Model file for the job. Use its own axes, mm. Face numbers are marked on the shaded views. A direction names the side the tool comes from. Round coordinates to 2 decimals unless told otherwise and drop trailing zeros. Loops run counter-clockwise (first coordinate to the right, second up) from the corner with the lowest first, then second, coordinate; pieces in that order, holes last. Notation, with made-up numbers: M 64.5,39 L 105.5,39 A15 ccw 105.5,64 Z; hole C 34.25,25.5 d8. An arc over 180 degrees is marked long. Use a Markdown table: item, result. Add a question column.
Item 1: Saw through at A-A on z = 1.5. Write the cut outline in (x, y), then the cut area to 3 significant figures.
Item 2: Wall check: L1, parallel to Z at x = -16.5, y = 11; L2, parallel to X at y = -15, z = 12.5; L3, parallel to X at y = -8, z = 24.5. Give the ranges that are in metal, low to high. Write a range as from..to.
Item 3: Tool access for the marked faces 1, 2 and 3: list every direction of +Z, -Z, +X, -X, +Y, -Y with a clear straight run to the whole face (end or side of a thin tool).
Item 4: Saw through at C-C on x = 0. Write the cut outline in (y, z), then the cut area to 3 significant figures.
Item 5: Pin check, flat tips, straight feed: P1, Ø8, axis at x = -2, y = -15, coming from the +Z side; P2, Ø4, axis at x = -23.5, z = 15.5, coming from the +Y side; P3, Ø2, axis at x = 1, z = 6, coming from the +Y side. Stop position of each tip, or through.
Item 6: Saw through at D-D on y = -4. Write the cut outline in (x, z).
Item 7: Two-plate mould, pull along X, no slides. Class the marked faces 4, 5, 6 and 7: +X half, -X half, draft (parallel to the pull), parting line (faces both ways), or undercut.
Item 8: Saw through at B-B on y = 15. Write the cut outline in (x, z).
```python
from build123d import *

# Parameters (mm, degrees)
F1_DEPTH = 6.604
F3_DEPTH = 19.05
F4_DEPTH = 25.4


with BuildPart() as f1:
    # F0 (on Top) → F1 (new body)
    with BuildSketch(Plane.XY):
        with BuildLine():
            ThreePointArc((31.75, 12.954), (29.9645229381, 17.2645229381), (25.654, 19.05))
            Line((25.654, 19.05), (-25.654, 19.05))
            ThreePointArc((-25.654, 19.05), (-29.9645229381, 17.2645229381), (-31.75, 12.954))
            Line((-31.75, 12.954), (-31.75, -19.05))
            Line((-31.75, -19.05), (31.75, -19.05))
            Line((31.75, -19.05), (31.75, 12.954))
        make_face()
    extrude(amount=F1_DEPTH)

    # F2 (on face) → F3 (join)
    with BuildSketch(Plane.XY.offset(6.604)):
        with BuildLine():
            Line((-25.4, -19.05), (-18.796, -19.05))
            Line((-18.796, -19.05), (-18.796, -8.7467487901))
            Line((-18.796, -8.7467487901), (0, -8.7467487901))
            Line((0, -8.7467487901), (18.796, -8.7467487901))
            Line((18.796, -8.7467487901), (18.796, -19.05))
            Line((18.796, -19.05), (25.4, -19.05))
            Line((25.4, -19.05), (25.4, 0))
            Line((25.4, 0), (21.844, 0))
            ThreePointArc((21.844, 0), (17.174266817, 1.934266817), (15.24, 6.604))
            Line((15.24, 6.604), (15.24, 19.05))
            Line((15.24, 19.05), (11.43, 19.05))
            ThreePointArc((11.43, 19.05), (0, 8.0444168312), (-11.43, 19.05))
            Line((-11.43, 19.05), (-15.24, 19.05))
            Line((-15.24, 19.05), (-15.24, 6.604))
            ThreePointArc((-15.24, 6.604), (-17.174266817, 1.934266817), (-21.844, 0))
            Line((-21.844, 0), (-25.4, 0))
            Line((-25.4, 0), (-25.4, -19.05))
        make_face()
    extrude(amount=F3_DEPTH)

    # F4 (cut): a face of the model
    f4_faces = [f1.faces().sort_by_distance(p)[0] for p in [
        (0, 14.3934898102, 6.604),
    ]]
    extrude(f4_faces, amount=-F4_DEPTH, mode=Mode.SUBTRACT)


solid = f1.part
```
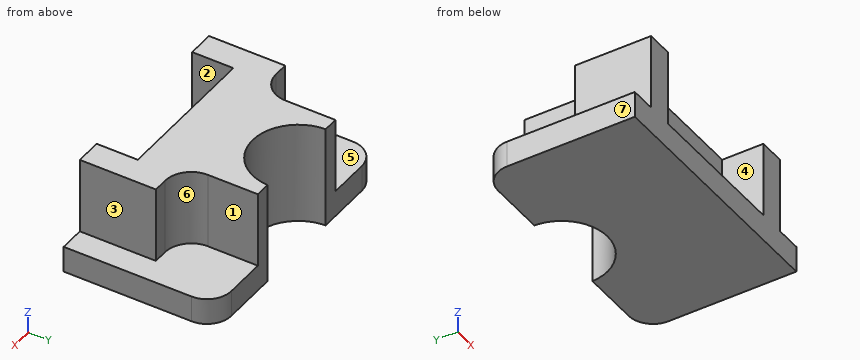
Entries:
| question | item | result |
|---|---|---|
| 1 | outline | M -31.75,-19.05 L 31.75,-19.05 L 31.75,12.95 A6.1 ccw 25.65,19.05 L 11.43,19.05 A11.44 cw -11.43,19.05 L -25.65,19.05 A6.1 ccw -31.75,12.95 Z |
| 1 | area | 2,210 mm2 |
| 2 | L1 | 0..6.6 |
| 2 | L2 | -25.4..-18.8, 18.8..25.4 |
| 2 | L3 | -25.4..25.4 |
| 3 | face 1 | +Z, +X, +Y |
| 3 | face 2 | +Z, -Y |
| 3 | face 3 | +Z, +X, +Y, -Y |
| 4 | outline | M -19.05,0 L 8.04,0 L 8.04,25.65 L -8.75,25.65 L -8.75,6.6 L -19.05,6.6 Z |
| 4 | area | 499 mm2 |
| 5 | P1 | z = 6.6 |
| 5 | P2 | y = 0.01 |
| 5 | P3 | y = 8.22 |
| 6 | outline | M -31.75,0 L 31.75,0 L 31.75,6.6 L 25.4,6.6 L 25.4,25.65 L -25.4,25.65 L -25.4,6.6 L -31.75,6.6 Z |
| 7 | face 4 | undercut |
| 7 | face 5 | draft |
| 7 | face 6 | +X half |
| 7 | face 7 | -X half |
| 8 | outline | M -31.4,0 L -10.52,0 L -10.52,25.65 L -15.24,25.65 L -15.24,6.6 L -31.4,6.6 Z; M 10.52,0 L 31.4,0 L 31.4,6.6 L 15.24,6.6 L 15.24,25.65 L 10.52,25.65 Z |
